```python
from build123d import *

# Parameters (mm, degrees)
SKETCH_1_R          = 3.3
EXTRUDE_1_DEPTH     = 26
CHAMFER_1_SIZE      = 3
SKETCH_2_R          = 7
CUT_EXTRUDE_1_DEPTH = 12
SKETCH_3_R          = 4.5
CUT_EXTRUDE_2_DEPTH = 64.686733312


with BuildPart() as part:
    # 草图1 → 凸台-拉伸1 (new body)
    # profile 1 of 2: a face of its own
    with BuildSketch(Plane(origin=(0, 0, 0), x_dir=(1, 0, 0), z_dir=(0, 1, 0))):
        with BuildLine():
            Line((0, 19), (0, 35))
            Line((0, 35), (-26, 35))
            Line((-26, 35), (-26, 25))
            Line((-26, 25), (-44, 25))
            Line((-44, 25), (-44, -25))
            Line((-44, -25), (0, -25))
            Line((0, -25), (0, -1))
            ThreePointArc((0, -1), (-10, 9), (0, 19))
        make_face()
        with Locations(Location((-35, -13, 0), (0, 0, 90))):
            Circle(SKETCH_1_R, mode=Mode.SUBTRACT)
        with Locations(Location((-35, 9, 0), (0, 0, 90))):
            Circle(SKETCH_1_R, mode=Mode.SUBTRACT)
    # profile 2 of 2: a face of its own
    with BuildSketch(Plane(origin=(0, 0, 0), x_dir=(1, 0, 0), z_dir=(0, 1, 0))):
        with BuildLine():
            Line((26, 35), (0, 35))
            Line((0, 35), (0, 19))
            ThreePointArc((0, 19), (7.071067812, 16.071067812), (10, 9))
            ThreePointArc((10, 9), (7.071067812, 1.928932188), (0, -1))
            Line((0, -1), (0, -25))
            Line((0, -25), (44, -25))
            Line((44, -25), (44, 25))
            Line((44, 25), (26, 25))
            Line((26, 25), (26, 35))
        make_face()
        with Locations(Location((35, -13, 0), (0, 0, 90))):
            Circle(SKETCH_1_R, mode=Mode.SUBTRACT)
        with Locations(Location((35, 9, 0), (0, 0, 90))):
            Circle(SKETCH_1_R, mode=Mode.SUBTRACT)
    extrude(amount=EXTRUDE_1_DEPTH)

    # 倒角1
    chamfer_1_edges = [part.edges().sort_by_distance(p)[0] for p in [
        (-26, 13, -35),
        (26, 13, -35),
    ]]
    chamfer(chamfer_1_edges, length=CHAMFER_1_SIZE)

    # 草图2 → 切除-拉伸1 (cut)
    with BuildSketch(Plane(origin=(0, 0, -25), x_dir=(-1, 0, 0), z_dir=(0, 0, -1))):
        with Locations((-35, 13)):
            Circle(SKETCH_2_R)
        with Locations(Location((35, 13, 0), (0, 0, 180))):
            Circle(SKETCH_2_R)
    extrude(amount=-CUT_EXTRUDE_1_DEPTH, mode=Mode.SUBTRACT)

    # 草图3 → 切除-拉伸2 (cut, through all)
    with BuildSketch(Plane(origin=(0, 0, -13), x_dir=(-1, 0, 0), z_dir=(0, 0, -1))):
        with Locations((-35, 13)):
            Circle(SKETCH_3_R)
        with Locations((35, 13)):
            Circle(SKETCH_3_R)
    extrude(amount=-CUT_EXTRUDE_2_DEPTH, mode=Mode.SUBTRACT)


solid = part.part
```
Model file for the job. Use its own axes, mm. A direction names the side the tool comes from. Coordinates: 2 decimals unless noted, no trailing zeros. Loops run counter-clockwise (first coordinate to the right, second up) from the corner with the lowest first, then second, coordinate; pieces in that order, holes last. Notation, with made-up numbers: (46.5, -9.75) -> (54.5, -9.75) arc R30 ccw to (54.5, 25.25) -> close; hole circle Ø9 at (28.5, -1.75). An arc over 180 degrees is marked (long way). Answer as a JSON object with one key per item and string values.
Q1. Cut at B-B (y = 4). List the corners of the cut face in (x, z).
Report:
{"outline": "(-44, -25) -> (-26, -25) -> (-26, -32) -> (-23, -35) -> (23, -35) -> (26, -32) -> (26, -25) -> (44, -25) -> (44, 25) -> (-44, 25) -> close; hole circle Ø6.6 at (-35, -9); hole circle Ø6.6 at (-35, 13); hole circle Ø20 at (0, -9); hole circle Ø6.6 at (35, -9); hole circle Ø6.6 at (35, 13)"}
Q2. Flat gauge pins, fed straight in: P1, Ø5.5, axis at x = -37.5, y = 12.5, coming from the -Z side; P2, Ø8.5, axis at x = 35, z = 13, coming from the +Y side; P3, Ø7.5, axis at y = 7, z = -29, coming from the -X side; P4, Ø8.5, axis at x = 35, y = 13, coming from the +Z side. Where does each tip first touch, or does it go through?
Report:
{"P1": "stops at z = -13", "P2": "stops at y = 26", "P3": "stops at x = -26", "P4": "passes through"}
Q3. Cut at D-D (x = -35). List the corners of the cut face in (y, z), and give its area (3 significant figures).
Report:
{"outline": "(0, -25) -> (6, -25) -> (6, -13) -> (8.5, -13) -> (8.5, -12.3) -> (0, -12.3) -> close; (0, -5.7) -> (8.5, -5.7) -> (8.5, 9.7) -> (0, 9.7) -> close; (0, 16.3) -> (8.5, 16.3) -> (8.5, 25) -> (0, 25) -> close; (17.5, -13) -> (20, -13) -> (20, -25) -> (26, -25) -> (26, -12.3) -> (17.5, -12.3) -> close; (17.5, -5.7) -> (26, -5.7) -> (26, 9.7) -> (17.5, 9.7) -> close; (17.5, 16.3) -> (26, 16.3) -> (26, 25) -> (17.5, 25) -> close", "area": "566 mm2"}
Q4. Cut at C-C (x = -5). List the corners of the cut face in (y, z).
Report:
{"outline": "(0, -35) -> (26, -35) -> (26, -17.66) -> (0, -17.66) -> close; (0, -0.34) -> (26, -0.34) -> (26, 25) -> (0, 25) -> close"}
Q5. Cut at A-A (y = 13). List the corners of the cut face in (x, z), and give its area (3 significant figures).
Report:
{"outline": "(-44, -25) -> (-42, -25) -> (-42, -13) -> (-39.5, -13) -> (-39.5, 25) -> (-44, 25) -> close; (-30.5, -13) -> (-28, -13) -> (-28, -25) -> (-26, -25) -> (-26, -32) -> (-23, -35) -> (23, -35) -> (26, -32) -> (26, -25) -> (28, -25) -> (28, -13) -> (30.5, -13) -> (30.5, 25) -> (-30.5, 25) -> close; (39.5, -13) -> (42, -13) -> (42, -25) -> (44, -25) -> (44, 25) -> (39.5, 25) -> close; hole circle Ø20 at (0, -9)", "area": "3,580 mm2"}
Q6. Pull direction Y, two halves, no side cores. Call faces 4 (the flat face through (35, 8, -13)), 5 (the flat face through (-0.6, 26, 1.2)), 6 (the flat face through (-39, 7, -25)): released by +Y, released by -Y, zero draft, split by the parting line, or undercut.
Report:
{"face 4": "undercut", "face 5": "released by +Y", "face 6": "zero draft"}
Q7. 3-axis set-ups, long thin cutter, end or side, ignore diameter. For faces 1 (the flat face through (26, 13, -28)), 2 (the cylindrical face through (-28.534, 15.681, -19.084)), 3 (the flat face through (-26, 13, -29)): which of +Z, -Z, +X, -X, +Y, -Y reach the whole face in a straight line?
Report:
{"face 1": "-Z, +X, +Y, -Y", "face 2": "-Z", "face 3": "-Z, -X, +Y, -Y"}
Q8. Probe probe 1 along X at (y, z) = (3.75, -9); probe 2 along X at (y, z) = (2, 13); probe 3 along Z at (x, y) = (-35, 20.5). List the from-to ranges inside material, lowest first.
Report:
{"probe 1": "x = -44 to -38.3, -31.7 to -10, 10 to 31.7, 38.3 to 44", "probe 2": "x = -44 to -38.3, -31.7 to 31.7, 38.3 to 44", "probe 3": "z = -25 to -12.3, -5.7 to 9.7, 16.3 to 25"}
